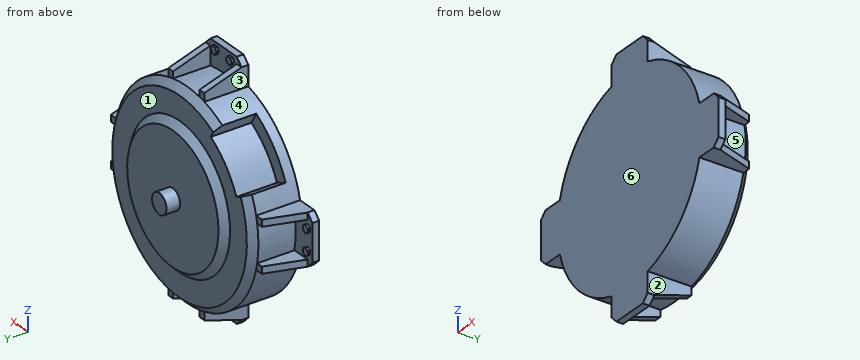
```python
from build123d import *

# Parameters (mm, degrees)
SKETCH1_R                    = 150
BOSS_EXTRUDE1_DEPTH          = 75
CHAMFER1_SIZE                = 10
BOSS_EXTRUDE2_DEPTH          = 10
CHAMFER2_SIZE                = 10
BOSS_EXTRUDE3_DEPTH          = 10
BOSS_EXTRUDE4_DEPTH          = 3.5
CIRPATTERN1_COUNT            = 4
CIRPATTERN1_COPY_1_DEPTH     = 10
CIRPATTERN1_COPY_2_DEPTH     = 10
CIRPATTERN1_COPY_3_DEPTH     = 10
CIRPATTERN1_COPY_4_DEPTH     = 3.5
CIRPATTERN1_COPY_5_DEPTH     = 3.5
CIRPATTERN1_COPY_6_DEPTH     = 3.5
CHAMFER2_OF_CIRPATTERN1_SIZE = 10
CUT_EXTRUDE2_START           = -60
CUT_EXTRUDE2_DEPTH           = 60
SKETCH6_R                    = 110
BOSS_EXTRUDE5_DEPTH          = 10
CHAMFER3_SIZE                = 15
SKETCH7_R                    = 15
BOSS_EXTRUDE6_DEPTH          = 20


with BuildPart() as part:
    # Sketch1 → Boss-Extrude1 (new body)
    with BuildSketch(Plane(origin=(0, 0, 0), x_dir=(1, 0, 0), z_dir=(0, 1, 0))):
        with Locations(Location((0, 0, 0), (0, 0, 270))):
            Circle(SKETCH1_R)
    extrude(amount=BOSS_EXTRUDE1_DEPTH)

    # Chamfer1
    chamfer1_edges = [part.edges().sort_by_distance(p)[0] for p in [
        (0, 75, -150),
    ]]
    chamfer(chamfer1_edges, length=CHAMFER1_SIZE)

    # Sketch2 → Boss-Extrude2 (add)
    with BuildSketch(Plane.XZ):
        with BuildLine():
            Line((-145.236875483, 37.5), (-185, 37.5))
            Line((-185, 37.5), (-185, -37.5))
            Line((-185, -37.5), (-145.236875483, -37.5))
            ThreePointArc((-145.236875483, -37.5), (-150, 0), (-145.236875483, 37.5))
        make_face()
    boss_extrude2 = extrude(amount=-BOSS_EXTRUDE2_DEPTH)

    # Chamfer2
    chamfer2_edges = [part.edges().sort_by_distance(p)[0] for p in [
        (-185, 5, -37.5),
        (-185, 5, 37.5),
    ]]
    chamfer(chamfer2_edges, length=CHAMFER2_SIZE)

    # Sketch3 → Boss-Extrude3 (add)
    with BuildSketch(Plane.XY.offset(37.5)):
        Polygon((-145.236875483, 10), (-145.236875483, 65), (-157.32, 65), (-175, 10), align=None)
    boss_extrude3 = extrude(amount=-BOSS_EXTRUDE3_DEPTH)

    # Sketch4 → Boss-Extrude4 (add)
    with BuildSketch(Plane(origin=(0, 10, 0), x_dir=(1, 0, 0), z_dir=(0, 1, 0))):
        Polygon((-175, -21.74912957), (-169.803847577, -18.74912957), (-169.803847577, -12.74912957), (-175, -9.74912957), (-180.196152423, -12.74912957), (-180.196152423, -18.74912957), align=None)
    boss_extrude4 = extrude(amount=BOSS_EXTRUDE4_DEPTH)

    # Mirror1: Boss-Extrude3, Boss-Extrude4 across plane
    add(boss_extrude3.mirror(Plane.XY))
    add(boss_extrude4.mirror(Plane.XY))

    # CirPattern1: Boss-Extrude2, Boss-Extrude3, Boss-Extrude4 ×4 about axis
    cirpattern1_axis = Axis((0, 0, 0), (0, 1, 0))
    add([boss_extrude2.rotate(cirpattern1_axis, i * 360 / CIRPATTERN1_COUNT) for i in range(1, CIRPATTERN1_COUNT)])
    add([boss_extrude3.rotate(cirpattern1_axis, i * 360 / CIRPATTERN1_COUNT) for i in range(1, CIRPATTERN1_COUNT)])
    add([boss_extrude4.rotate(cirpattern1_axis, i * 360 / CIRPATTERN1_COUNT) for i in range(1, CIRPATTERN1_COUNT)])

    # CirPattern1 copy 1 sketch → CirPattern1 copy 1 (add)
    with BuildSketch(Plane(origin=(-37.5, 0, 0), x_dir=(0, 0, -1), z_dir=(-1, 0, 0))):
        Polygon((-145.236875483, -10), (-145.236875483, -65), (-157.32, -65), (-175, -10), align=None)
    extrude(amount=-CIRPATTERN1_COPY_1_DEPTH)

    # CirPattern1 copy 2 sketch → CirPattern1 copy 2 (add)
    with BuildSketch(Plane(origin=(0, 0, 37.5), x_dir=(-1, 0, 0), z_dir=(0, 0, 1))):
        Polygon((-145.236875483, -10), (-145.236875483, -65), (-157.32, -65), (-175, -10), align=None)
    extrude(amount=-CIRPATTERN1_COPY_2_DEPTH)

    # CirPattern1 copy 3 sketch → CirPattern1 copy 3 (add)
    with BuildSketch(Plane(origin=(37.5, 0, 0), x_dir=(0, 0, 1), z_dir=(1, 0, 0))):
        Polygon((-145.236875483, -10), (-145.236875483, -65), (-157.32, -65), (-175, -10), align=None)
    extrude(amount=-CIRPATTERN1_COPY_3_DEPTH)

    # CirPattern1 copy 4 sketch → CirPattern1 copy 4 (add)
    with BuildSketch(Plane(origin=(0, 10, 0), x_dir=(0, 0, -1), z_dir=(0, 1, 0))):
        Polygon((-175, 21.74912957), (-169.803847577, 18.74912957), (-169.803847577, 12.74912957), (-175, 9.74912957), (-180.196152423, 12.74912957), (-180.196152423, 18.74912957), align=None)
    extrude(amount=CIRPATTERN1_COPY_4_DEPTH)

    # CirPattern1 copy 5 sketch → CirPattern1 copy 5 (add)
    with BuildSketch(Plane(origin=(0, 10, 0), x_dir=(-1, 0, 0), z_dir=(0, 1, 0))):
        Polygon((-175, 21.74912957), (-169.803847577, 18.74912957), (-169.803847577, 12.74912957), (-175, 9.74912957), (-180.196152423, 12.74912957), (-180.196152423, 18.74912957), align=None)
    extrude(amount=CIRPATTERN1_COPY_5_DEPTH)

    # CirPattern1 copy 6 sketch → CirPattern1 copy 6 (add)
    with BuildSketch(Plane.ZX.offset(10)):
        Polygon((-175, 21.74912957), (-169.803847577, 18.74912957), (-169.803847577, 12.74912957), (-175, 9.74912957), (-180.196152423, 12.74912957), (-180.196152423, 18.74912957), align=None)
    extrude(amount=CIRPATTERN1_COPY_6_DEPTH)

    # Chamfer2 of CirPattern1
    chamfer2_of_cirpattern1_edges = [part.edges().sort_by_distance(p)[0] for p in [
        (-37.5, 5, 185),
        (37.5, 5, 185),
        (185, 5, 37.5),
        (185, 5, -37.5),
        (37.5, 5, -185),
        (-37.5, 5, -185),
    ]]
    chamfer(chamfer2_of_cirpattern1_edges, length=CHAMFER2_OF_CIRPATTERN1_SIZE)

    # Sketch5 → Cut-Extrude2 (cut)
    with BuildSketch(Plane(origin=(0, 75, 0), x_dir=(1, 0, 0), z_dir=(0, 1, 0)).offset(CUT_EXTRUDE2_START)):
        with BuildLine():
            ThreePointArc((-70, -121.24355653), (-103.548353297, -94.221751891), (-127.293055267, -58.279310916))
            Line((-127.293055267, -58.279310916), (-136.385416357, -62.442118839))
            ThreePointArc((-136.385416357, -62.442118839), (-110.944664247, -100.951877026), (-75, -129.903810568))
            Line((-75, -129.903810568), (-70, -121.24355653))
        make_face()
        with BuildLine():
            ThreePointArc((-65, -112.583302492), (-96.152042347, -87.491626756), (-118.200694176, -54.116502994))
            Line((-118.200694176, -54.116502994), (-127.293055267, -58.279310916))
            ThreePointArc((-127.293055267, -58.279310916), (-103.548353297, -94.221751891), (-70, -121.24355653))
            Line((-70, -121.24355653), (-65, -112.583302492))
        make_face()
    extrude(amount=CUT_EXTRUDE2_DEPTH, mode=Mode.SUBTRACT)

    # Sketch6 → Boss-Extrude5 (add)
    with BuildSketch(Plane(origin=(0, 75, 0), x_dir=(1, 0, 0), z_dir=(0, 1, 0))):
        with Locations(Location((0, 0, 0), (0, 0, 270))):
            Circle(SKETCH6_R)
    extrude(amount=BOSS_EXTRUDE5_DEPTH)

    # Chamfer3
    # the kernel refuses this chamfer: 15 mm, written as the material it takes off along each edge
    with BuildSketch(Plane(origin=(0, 85, 0), x_dir=(0, 0, 1), z_dir=(-1, 0, 0))) as chamfer3_piece_1_section:
        Polygon((110, -CHAMFER3_SIZE), (110 - CHAMFER3_SIZE, 0), (110, 0), align=None)
    chamfer3_piece_1 = revolve(axis=Axis((0, 85, 0), (0, 1, 0)), mode=Mode.PRIVATE)
    chamfer3_piece_1 = split(chamfer3_piece_1, bisect_by=Plane(origin=(0, 75, -100.081022807), z_dir=(0, 1, 0)), keep=Keep.TOP, mode=Mode.PRIVATE)
    add(chamfer3_piece_1, mode=Mode.SUBTRACT)

    # Sketch7 → Boss-Extrude6 (add)
    with BuildSketch(Plane(origin=(0, 85, 0), x_dir=(1, 0, 0), z_dir=(0, 1, 0))):
        with Locations(Location((0, 0, 0), (0, 0, 270))):
            Circle(SKETCH7_R)
    extrude(amount=BOSS_EXTRUDE6_DEPTH)


solid = part.part
```
The model under review builds one solid part; all positions refer to its coordinate system, in mm. Face numbers are marked on the shaded views. A direction names the side the tool comes from. Round coordinates to 2 decimals unless told otherwise and drop trailing zeros. Order: outer loops, then holes, each group sorted by start corner. A loop starts at its lowest first (then second) coordinate and runs counter-clockwise, first axis right, second up. Notation, with made-up numbers: (10, -20) -> (43, -20) arc R22 cw to (43, -12) -> close; hole circle Ø9 at (27.5, 54). An arc over 180 degrees is marked (long way). One line per item, written item: value. Start each with the question number.
Q1. Mouldability with a two-part tool opening along Z and no side actions: class the marked faces 4, 5 and 6 as released by +Z, released by -Z, zero draft, split by the parting line, or undercut.
Q2. Take a section at A-A (x = 0). Write out the cut boundary in (y, z), and give its area (3 significant figures).
Q3. Clearance check with flat-ended pins moving along their axes: pin 1 Ø14 at (y, z) = (38.5, 154.5) entering from -X; pin 2 Ø1.8 at (y, z) = (12.5, 17) entering from -X; pin 3 Ø1.5 at (x, y) = (137.5, 32.5) entering from -Z. State where each tip first meets the part, or that it passes through.
Q4. Wall thickness on line 1 (Z direction, x = 151, y = 40.5); line 2 (Y direction, x = 35, z = -124): over which ranges is each line inside the solid? List them lowest first.
Q5. Machinability: for the marked faces 1, 2 and 3, which of the approach directions +Z, -Z, +X, -X, +Y, -Y give a long, thin tool a straight path to every point of the face, cutting with its end or side? Answer none if there is none.
Q6. Take a section at B-B (z = 0). Write out the cut boundary in (x, y).
Q7. Take a section at C-C (y = 97.5). Write out the cut boundary in (x, z), and give its area (3 significant figures).
Reported:
1. face 4: released by +Z
1. face 5: undercut
1. face 6: zero draft
2. outline: (0, -185) -> (10, -185) -> (10, -150) -> (65, -150) -> (75, -140) -> (75, -105) -> (85, -95) -> (85, -15) -> (105, -15) -> (105, 15) -> (85, 15) -> (85, 95) -> (75, 105) -> (75, 140) -> (65, 150) -> (10, 150) -> (10, 185) -> (0, 185) -> close
2. area: 25,700 mm2
3. pin 1: stops at x = -37.5
3. pin 2: stops at x = -180.2
3. pin 3: stops at z = -61.64
4. line 1: z = -37.5 to -27.5, 27.5 to 37.5
4. line 2: y = 0 to 75
5. face 1: +Y
5. face 2: -Z, +X, +Y, -Y
5. face 3: +Z, -X, +Y, -Y
6. outline: (-185, 0) -> (185, 0) -> (185, 10) -> (150, 10) -> (150, 65) -> (140, 75) -> (105, 75) -> (95, 85) -> (15, 85) -> (15, 105) -> (-15, 105) -> (-15, 85) -> (-95, 85) -> (-105, 75) -> (-140, 75) -> (-150, 65) -> (-150, 10) -> (-185, 10) -> close
7. outline: circle Ø30 at (0, 0)
7. area: 707 mm2
